Can you work these out from the model? Positions are in its coordinate system, mm. A direction names the side the tool comes from. Round coordinates to 2 decimals unless told otherwise and drop trailing zeros. Loops run counter-clockwise (first coordinate to the right, second up) from the corner with the lowest first, then second, coordinate; pieces in that order, holes last. Notation, with made-up numbers: (-34.5, -23.75) -> (22.5, -23.75) arc R21 cw to (22.5, 3.25) -> close; hole circle Ø4 at (63, 66.5). An arc over 180 degrees is marked (long way). Use a Markdown table: item, result.
Autodesk Inventor part; units mm, degrees
ref_plane "YZ Plane" through (0, 0, 0) normal (1, 0, 0) x (0, 1, 0)
ref_plane "XZ Plane" through (0, 0, 0) normal (0, 1, 0) x (-1, 0, 0)
ref_plane "XY Plane" through (0, 0, 0) normal (0, 0, 1) x (1, 0, 0)
sketch "Sketch1" plane through (0, 0, 0) normal (1, 0, 0) x (0, 1, 0)
  arc A0 (14.7437, -9.9374) -> (-14.7437, -9.9374) centre (0, 0) ccw
  arc A1 (-8.382, -127) -> (8.382, -127) centre (0, -127) ccw
  line L0 (-3.2996, -10.4245) -> (-7.3781, -8.0697)
  line L1 (-10.6776, -2.3547) -> (-10.6776, 2.3547)
  line L2 (-7.3781, 8.0697) -> (-3.2996, 10.4245)
  line L3 (3.2996, 10.4245) -> (7.3781, 8.0697)
  line L4 (10.6776, 2.3547) -> (10.6776, -2.3547)
  line L5 (7.3781, -8.0697) -> (3.2996, -10.4245)
  arc A2 (10.6776, 2.3547) -> (7.3781, 8.0697) centre (7.3781, 4.2597) ccw
  arc A3 (7.3781, -8.0697) -> (10.6776, -2.3547) centre (7.3781, -4.2597) ccw
  arc A4 (3.2996, 10.4245) -> (-3.2996, 10.4245) centre (0, 8.5195) ccw
  arc A5 (-7.3781, 8.0697) -> (-10.6776, 2.3547) centre (-7.3781, 4.2597) ccw
  arc A6 (-10.6776, -2.3547) -> (-7.3781, -8.0697) centre (-7.3781, -4.2597) ccw
  arc A7 (-3.2996, -10.4245) -> (3.2996, -10.4245) centre (0, -8.5195) ccw
  line L6 (-3.2996, -73.9245) -> (-7.3781, -71.5697)
  line L7 (-10.6776, -65.8547) -> (-10.6776, -61.1453)
  line L8 (-7.3781, -55.4303) -> (-3.2996, -53.0755)
  line L9 (3.2996, -53.0755) -> (7.3781, -55.4303)
  line L10 (10.6776, -61.1453) -> (10.6776, -65.8547)
  line L11 (7.3781, -71.5697) -> (3.2996, -73.9245)
  arc A8 (10.6776, -61.1453) -> (7.3781, -55.4303) centre (7.3781, -59.2403) ccw
  arc A9 (7.3781, -71.5697) -> (10.6776, -65.8547) centre (7.3781, -67.7597) ccw
  arc A10 (3.2996, -53.0755) -> (-3.2996, -53.0755) centre (0, -54.9805) ccw
  arc A11 (-7.3781, -55.4303) -> (-10.6776, -61.1453) centre (-7.3781, -59.2403) ccw
  arc A12 (-10.6776, -65.8547) -> (-7.3781, -71.5697) centre (-7.3781, -67.7597) ccw
  arc A13 (-3.2996, -73.9245) -> (3.2996, -73.9245) centre (0, -72.0195) ccw
  circle A14 centre (0, -127) radius 4.765
  arc A15 (14.268, -11.0656) -> (14.268, -52.4344) centre (113.7401, -31.75) ccw
  arc A16 (-14.268, -52.4344) -> (-14.268, -11.0656) centre (-113.7401, -31.75) ccw
  arc A17 (14.2667, -74.5446) -> (8.382, -127) centre (262.3746, -128.9362) ccw
  arc A18 (-8.382, -127) -> (-14.2667, -74.5446) centre (-262.3746, -128.9362) ccw
  arc A19 (14.7365, -73.4481) -> (14.7437, -53.5626) centre (0, -63.5) ccw
  arc A20 (-14.7437, -53.5626) -> (-14.7365, -73.4481) centre (0, -63.5) ccw
  arc A21 (14.7365, -73.4481) -> (14.2667, -74.5446) centre (17.368, -75.2245) ccw
  arc A22 (14.268, -52.4344) -> (14.7437, -53.5626) centre (17.3765, -51.788) ccw
  arc A23 (-14.7437, -53.5626) -> (-14.268, -52.4344) centre (-17.3765, -51.788) ccw
  arc A24 (-14.2667, -74.5446) -> (-14.7365, -73.4481) centre (-17.368, -75.2245) ccw
  arc A25 (-14.268, -11.0656) -> (-14.7437, -9.9374) centre (-17.3765, -11.712) ccw
  arc A26 (14.7437, -9.9374) -> (14.268, -11.0656) centre (17.3765, -11.712) ccw
  dimension "d0" = 35.56
  dimension "d21" = 16.764
  dimension "d34" = 9.5301
  dimension "d35" = 101.6
  dimension "d36" = 101.6
  dimension "d37" = 254
  dimension "d38" = 254
  dimension "d39" = 3.175
extrude "Extrusion1" add sketch "Sketch1" along normal blind 15.24
properties part number "Kevin_CAD_test"
1. I want a section at B-B (z = 0). Please give me the cut outline in (x, y).
Answer sheet:
| item | result |
|---|---|
| outline | (0, -17.78) -> (15.24, -17.78) -> (15.24, -10.68) -> (0, -10.68) -> close; (0, 10.68) -> (15.24, 10.68) -> (15.24, 17.78) -> (0, 17.78) -> close |
2. If we mould it in two halves opening along Y, with no side actions, what happens to faces 3 (the flat face through (7.51, -5.37, 9.23)), 4 (the cylindrical face through (7.51, 0.18, -135.38)), 5 (the cylindrical face through (7.51, -17.78, -63.65))? For each: +Y half, -Y half, draft (parallel to the pull), parting line (faces both ways), or undercut.
Answer sheet:
| item | result |
|---|---|
| face 3 | undercut |
| face 4 | parting line |
| face 5 | -Y half |
3. I want a section at C-C (z = -64). Please give me the cut outline in (x, y).
Answer sheet:
| item | result |
|---|---|
| outline | (0, -17.77) -> (15.24, -17.77) -> (15.24, -10.68) -> (0, -10.68) -> close; (0, 10.68) -> (15.24, 10.68) -> (15.24, 17.77) -> (0, 17.77) -> close |
4. I want a section at A-A (y = 0). Please give me the cut outline in (x, z) (3 decimals).
Answer sheet:
| item | result |
|---|---|
| outline | (0, -135.382) -> (15.24, -135.382) -> (15.24, -131.765) -> (0, -131.765) -> close; (0, -122.235) -> (15.24, -122.235) -> (15.24, -75.83) -> (0, -75.83) -> close; (0, -51.17) -> (15.24, -51.17) -> (15.24, -12.33) -> (0, -12.33) -> close; (0, 12.33) -> (15.24, 12.33) -> (15.24, 17.78) -> (0, 17.78) -> close |
5. I want a section at D-D (x = 7.5). State how many separate pieces and enclosed holes the cut face has, plus the area to 3 significant figures.
Answer sheet:
| item | result |
|---|---|
| separate pieces | 1 |
| enclosed holes | 3 |
| area | 2,970 mm² |
6. I need wall thicknesses on line 1 (Y direction, x = 1.25, z = 1); line 2 (Z direction, x = 2.75, y = -3); line 3 (Y direction, x = 11, z = -12). Which ranges of each line are inside material? Lowest first, please.
Answer sheet:
| item | result |
|---|---|
| line 1 | y = -17.75 to -10.68, 10.68 to 17.75 |
| line 2 | z = -134.83 to -130.7, -123.3 to -74.37, -52.63 to -10.87, 10.87 to 17.53 |
| line 3 | y = -14.08 to -1.55, 1.55 to 14.08 |
7. Will these pins go through, and if not, where does the flat tip stop? pin 1 Ø5 at (x, y) = (11.5, -7.5) entering from +Z; pin 2 Ø5 at (x, z) = (10.5, -114.5) entering from -Y; pin 3 Ø1.4 at (x, z) = (8, -62.5) entering from +Y.
Answer sheet:
| item | result |
|---|---|
| pin 1 | stops at z = 17.06 |
| pin 2 | stops at y = -8.94 |
| pin 3 | stops at y = 17.78 |
8. Which directions (+Z, -Z, +X, -X, +Y, -Y) give clear straight access to the entire face, cutting with the end or side of a thin tool? Please do faces 1 (the flat face through (7.51, 5.37, -72.73)), 2 (the flat face through (0, 0, -41)).
Answer sheet:
| item | result |
|---|---|
| face 1 | +X, -X |
| face 2 | +Z, -Z, -X, +Y, -Y |
